Can you work these out from the model? Positions are in its coordinate system, mm. Face numbers are marked on the shaded views. A direction names the side the tool comes from. Give positions to 0.01 mm unless a question says otherwise; leave off trailing zeros. Order: outer loops, then holes, each group sorted by start corner. A loop starts at its lowest first (then second) coordinate and runs counter-clockwise, first axis right, second up. Notation, with made-up numbers: M 29.25,52.25 L 51.25,52.25 A20 ccw 51.25,82.25 Z; hole C 83.25,-14 d11. An arc over 180 degrees is marked long. Write each question's results on one line, items separated by ' | '.
from build123d import *

# Parameters (mm, degrees)
EXTRUDE_1_DEPTH     = 42
SKETCH_2_R          = 15
CUT_EXTRUDE_1_DEPTH = 12
SKETCH_3_W          = 30
SKETCH_3_H          = 20
CUT_EXTRUDE_2_DEPTH = 8
SKETCH_4_W          = 5
SKETCH_4_H          = 8
EXTRUDE_2_DEPTH     = 3
OTHER_START         = 8
OTHER_1_OUTLINE_R   = 1.7
OTHER_1_DEPTH       = 34
SKETCH_7_W          = 20
SKETCH_7_H          = 32
CUT_EXTRUDE_6_DEPTH = 26
CUT_EXTRUDE_7_DEPTH = 60.699246226


# Read off the part's stored shape, not the designer's step: 高级异型孔1
with BuildPart() as part:
    # 草图1 → 凸台-拉伸1 (new body)
    with BuildSketch(Plane.XY):
        with BuildLine():
            Line((0, 0), (5.769230769, -13.846153846))
            ThreePointArc((5.769230769, -13.846153846), (15, -20), (24.230769231, -13.846153846))
            Line((24.230769231, -13.846153846), (30, 0))
            Line((30, 0), (30, 30))
            Line((30, 30), (0, 30))
            Line((0, 30), (0, 0))
        make_face()
    extrude(amount=EXTRUDE_1_DEPTH)

    # 草图2 → 切除-拉伸1 (cut, symmetric)
    with BuildSketch(Plane(origin=(0, 0, 25), x_dir=(-1, 0, 0), z_dir=(0, 0, -1))):
        with Locations((-15, -10)):
            Circle(SKETCH_2_R)
    extrude(amount=CUT_EXTRUDE_1_DEPTH, both=True, mode=Mode.SUBTRACT)

    # 草图3 → 切除-拉伸2 (cut)
    with BuildSketch(Plane(origin=(0, 0, 0), x_dir=(-1, 0, 0), z_dir=(0, 0, -1))):
        with Locations((-15, -10)):
            Rectangle(SKETCH_3_W, SKETCH_3_H)
    extrude(amount=-CUT_EXTRUDE_2_DEPTH, mode=Mode.SUBTRACT)

    # 草图4 → 凸台-拉伸2 (add)
    with BuildSketch(Plane(origin=(0, 0, 0), x_dir=(-1, 0, 0), z_dir=(0, 0, -1))):
        with Locations((-27.5, 15)):
            Rectangle(SKETCH_4_W, SKETCH_4_H)
        with Locations((-2.5, 15)):
            Rectangle(SKETCH_4_W, SKETCH_4_H)
    extrude(amount=EXTRUDE_2_DEPTH)

    # 高级异型孔1 outline → 高级异型孔1 (cut)
    with BuildSketch(Plane.XY.offset(OTHER_START)):
        with Locations((15, -10)):
            Circle(OTHER_1_OUTLINE_R)
    extrude(amount=OTHER_1_DEPTH, mode=Mode.SUBTRACT)

    # 草图7 → 切除-拉伸6 (cut)
    with BuildSketch(Plane(origin=(0, 30, 0), x_dir=(1, 0, 0), z_dir=(0, 1, 0))):
        with Locations((15, -26)):
            Rectangle(SKETCH_7_W, SKETCH_7_H)
    extrude(amount=-CUT_EXTRUDE_6_DEPTH, mode=Mode.SUBTRACT)

    # 草图8 → 切除-拉伸7 (cut, through all)
    with BuildSketch(Plane(origin=(30, 0, 0), x_dir=(0, 0, -1), z_dir=(1, 0, 0))):
        Polygon((-42, 30), (-10, 30), (-42, 4), align=None)
    extrude(amount=-CUT_EXTRUDE_7_DEPTH, mode=Mode.SUBTRACT)


solid = part.part
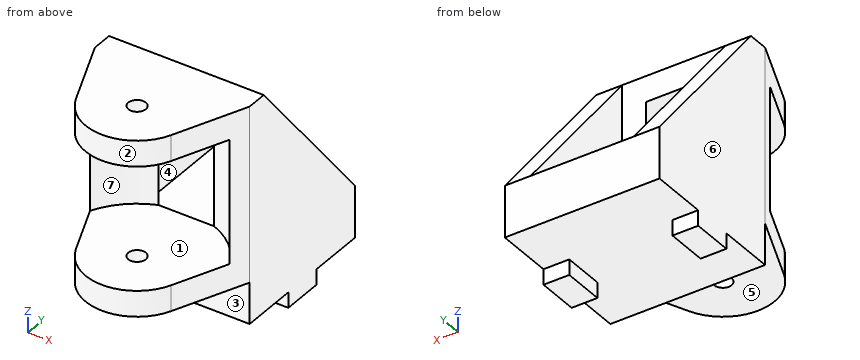
(1) We'd pull the mould along X, two halves only. Please class the marked faces 5, 6 and 7: +X half, -X half, draft (parallel to the pull), parting line (faces both ways), or undercut.
Data:
face 5: draft | face 6: -X half | face 7: undercut
(2) I need wall thicknesses on L1, parallel to X at y = 10, z = 29; L2, parallel to Z at x = 22.5, y = -4; L3, parallel to Y at x = 15, z = 40.35. Which ranges of each line are inside material? Lowest first, please. Write a range as from..to.
Data:
L1: x = 0..5, 25..30 | L2: z = 8..13, 37..42 | L3: y = -20..-11.7, -8.3..4
(3) Imagine slicing it at A-A, the plane z = 18. Write out the boundary of the cut face in (x, y), plus the area to 3 significant figures.
Data:
outline: M 0,0 L 1.47,-3.53 A15 cw 9.61,4 L 5,4 L 5,23.5 L 0,23.5 Z; M 20.39,4 A15 cw 28.53,-3.53 L 30,0 L 30,23.5 L 25,23.5 L 25,4 Z | area: 257 mm2
(4) Imagine slicing it at C-C, the plane z = 9. Write out the boundary of the cut face in (x, y), plus the area to 3 significant figures.
Data:
outline: M 0,0 L 5.77,-13.85 A10 ccw 24.23,-13.85 L 30,0 L 30,30 L 0,30 Z; hole C 15,-10 d3.4 | area: 1,310 mm2
(5) Imagine slicing it at D-D, the plane y = -10. Write out the boundary of the cut face in (x, z), plus the area to 3 significant figures.
Data:
outline: M 4.17,8 L 13.3,8 L 13.3,13 L 4.17,13 Z; M 4.17,37 L 13.3,37 L 13.3,42 L 4.17,42 Z; M 16.7,8 L 25.83,8 L 25.83,13 L 16.7,13 Z; M 16.7,37 L 25.83,37 L 25.83,42 L 16.7,42 Z | area: 183 mm2
(6) Imagine slicing it at B-B, the plane x = 15. Write out the boundary of the cut face in (y, z).
Data:
outline: M -20,8 L -11.7,8 L -11.7,13 L -20,13 Z; M -20,37 L -11.7,37 L -11.7,42 L -20,42 Z; M -8.3,8 L 0,8 L 0,0 L 30,0 L 30,10 L 4,10 L 4,13 L -8.3,13 Z; M -8.3,37 L 4,37 L 4,42 L -8.3,42 Z
(7) For the marked faces 1, 2, 3 and 4, which set-ups out of +Z, -Z, +X, -X, +Y, -Y let a thin tool reach every point of the face, with its end or its side?
Data:
face 1: -Y | face 2: +Z, -Z, -Y | face 3: -Z, +X, -X, -Y | face 4: +Z, +Y
(8) Will these pins go through, and if not, where does the flat tip stop? P1, Ø1.5, axis at x = 23.5, z = 25.5, coming from the -Y side; P2, Ø4.5, axis at x = 15, y = -10, coming from the -Z side; P3, Ø2.5, axis at x = 1.5, z = -1.5, coming from the -Y side; P4, Ø8, axis at y = 17.5, z = 33, coming from the +X side.
Data:
P1: stops at y = 1.81 | P2: stops at z = 8 | P3: stops at y = 11 | P4: passes through
